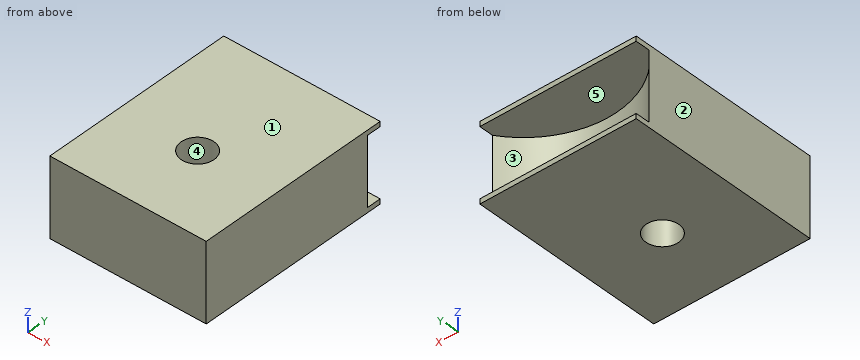
Autodesk Inventor part; units mm, degrees
ref_plane "YZ Plane" through (0, 0, 0) normal (1, 0, 0) x (0, 1, 0)
ref_plane "XZ Plane" through (0, 0, 0) normal (0, 1, 0) x (-1, 0, 0)
ref_plane "XY Plane" through (0, 0, 0) normal (0, 0, 1) x (1, 0, 0)
sketch "Sketch3" plane through (0, 0, 0) normal (0, 0, 1) x (1, 0, 0)
  line L0 (-12.7, -19.05) -> (12.7, -19.05)
  line L1 (12.7, -19.05) -> (12.7, 19.05)
  line L2 (12.7, 19.05) -> (-12.7, 19.05)
  line L3 (-12.7, 19.05) -> (-12.7, -19.05)
  line L4 (-12.7, -19.05) -> (12.7, 19.05) construction
  line L5 (12.7, -19.05) -> (-12.7, 19.05) construction
  point P0 (0, 0)
  dimension "d0" = 25.4
  dimension "d1" = 38.1
extrude "Extrusion1" add sketch "Sketch3" along normal mid plane 12.7
sketch "Sketch4" plane through (0, 0, 6.35) normal (0, 0, 1) x (1, 0, 0)
  circle A0 centre (0, 0) radius 2.667
  dimension "d4" = 5.334
extrude "Extrusion2" cut sketch "Sketch4" against normal through all
sketch "Sketch5" plane through (-12.7, -19.05, 6.35) normal (-1, 0, 0) x (0, 0, 1)
  line L0 (3.175, 6.35) -> (50.8, 6.35)
  line L1 (-12.7, 38.1) -> (-12.7, 0)
  line L2 (0, 0) -> (0, 38.1)
  line L3 (-12.7, 0) -> (0, 0)
  line L4 (0, 0) -> (0, 6.35)
  line L5 (0, 6.35) -> (-12.7, 6.35)
  line L6 (-12.7, 6.35) -> (-12.7, 0)
  point P0 (-6.35, 19.05)
  point P1 (-12.7, 6.35)
  dimension "d9" = 6.35
extrude "Extrusion3" cut sketch "Sketch5" against normal through all
sketch "Sketch6" plane through (0, 0, 0) normal (0, 0, 1) x (1, 0, 0)
  circle A0 centre (0, 25.4) radius 15.367
  point P0 (0, 0)
  dimension "d10" = 25.4
  dimension "d13" = 30.734
extrude "Extrusion4" cut sketch "Sketch6" along normal mid plane 11.0998
properties part number "preventWireJumping" material "PBT Plastic"
Input: part model. Units: mm. Frame: model coordinates. Face numbers are marked on the shaded views. A direction names the side the tool comes from. Round coordinates to 2 decimals unless told otherwise and drop trailing zeros. Loops run counter-clockwise (first coordinate to the right, second up) from the corner with the lowest first, then second, coordinate; pieces in that order, holes last. Notation, with made-up numbers: (54.5, 24) -> (92.5, 24) arc R17 ccw to (92.5, 56) -> close; hole circle Ø2 at (-20.5, 1). An arc over 180 degrees is marked (long way). Answer as a JSON object with one key per item and string values. Group by question number.
1) Ray query, L1, parallel to Z at x = -5.5, y = 16; L2, parallel to Y at x = 0, z = -3; L3, parallel to X at y = -0.5, z = -5.75. Return the intervals inside material, ascending.
2) Pin query (flat end, axial travel): pin 1 (5 mm diameter, centred on x = -1, z = -3, fed in from +Y); pin 2 (3 mm diameter, centred on x = 0, y = 0, fed in from +Z); pin 3 (4 mm diameter, centred on x = -4, z = 3, fed in from +Y). Return the tip coordinate at first contact, or that it passes through.
3) Draft query along Z for the marked faces 1, 2 and 3. Return one class per face: +Z half, -Z half, draft (parallel to the pull), parting line (faces both ways), or undercut.
4) Section query B-B on z = -2.75. Output: boundary loops of the cut face in (x, y).
5) Section query A-A on y = 0. Output: boundary loops of the cut face in (x, z), plus the area to 3 significant figures.
6) Reachability of the marked faces 4 and 5 from +Z, -Z, +X, -X, +Y, -Y: full face, straight path, thin tool, end or side. Return the list, or none.
7) Section query D-D on y = 13.5. Output: boundary loops of the cut face in (x, z), plus the area to 3 significant figures.
8) Section query C-C on x = 0. Output: boundary loops of the cut face in (y, z), plus the area to 3 significant figures.
Reply:
{
 "1": {"L1": "z = -6.35 to -5.55, 5.55 to 6.35", "L2": "y = -12.7 to -2.67, 2.67 to 10.03", "L3": "x = -12.7 to -2.62, 2.62 to 12.7"},
 "2": {"pin 1": "stops at y = 10.44", "pin 2": "passes through", "pin 3": "stops at y = 11.25"},
 "3": {"face 1": "+Z half", "face 2": "draft", "face 3": "undercut"},
 "4": {"outline": "(-12.7, -12.7) -> (12.7, -12.7) -> (12.7, 16.75) arc R15.37 cw to (-12.7, 16.75) -> close; hole circle Ø5.33 at (0, 0)"},
 "5": {"outline": "(-12.7, -6.35) -> (-2.67, -6.35) -> (-2.67, 6.35) -> (-12.7, 6.35) -> close; (2.67, -6.35) -> (12.7, -6.35) -> (12.7, 6.35) -> (2.67, 6.35) -> close", "area": "255 mm2"},
 "6": {"face 4": "+Z, -Z", "face 5": "+Y"},
 "7": {"outline": "(-12.7, -6.35) -> (12.7, -6.35) -> (12.7, 6.35) -> (-12.7, 6.35) -> close; hole (-9.72, -5.55) -> (9.72, -5.55) -> (9.72, 5.55) -> (-9.72, 5.55) -> close", "area": "107 mm2"},
 "8": {"outline": "(-12.7, -6.35) -> (-2.67, -6.35) -> (-2.67, 6.35) -> (-12.7, 6.35) -> close; (2.67, -6.35) -> (19.05, -6.35) -> (19.05, -5.55) -> (10.03, -5.55) -> (10.03, 5.55) -> (19.05, 5.55) -> (19.05, 6.35) -> (2.67, 6.35) -> close", "area": "235 mm2"}
}
